Verification items for the finished model (mm, model axes). A direction names the side the tool comes from. Give positions to 0.01 mm unless a question says otherwise; leave off trailing zeros. Write each loop counter-clockwise with the first axis right and the second up, starting at its lowest first coordinate (ties: lowest second). Pieces come first, ordered by that corner, then holes. Notation, with made-up numbers: (15, 13.25) -> (40, 13.25) arc R18 ccw to (40, 41.25) -> close; hole circle Ø10 at (72, 69.5). An arc over 180 degrees is marked (long way). Answer as CSV lines item,"result". Start each with the question number.
1) Gauge pin test, flat ends, axial feed: pin 1 Ø4 at (x, z) = (69, 22) entering from +Y; pin 2 Ø15 at (y, z) = (-137, 0.5) entering from -X; pin 3 Ø3 at (x, z) = (-3.5, 20.5) entering from +Y. Record the tip position at first contact, or that the pin passes through.
2) Sectioned sample at B-B on x = 118. Record the cut outline in (y, z), and give its area (3 significant figures).
3) Sectioned sample at A-A on z = -4.5. Record the cut outline in (x, y), and give its area (3 significant figures).
4) Material ranges on L1, parallel to Z at x = 101.5, y = -80; L2, parallel to X at y = -132.5, z = 8.5; L3, parallel to Y at x = 132, z = -8, recorded low to high.
5) Mould release check, pull along Z, two halves, no side actions. Record for faces 4 (the flat face through (0, -125, 8)), 5 (the flat face through (73.95, -134.863, 25.056)), 6 (the flat face through (125, -5, 17)): released by +Z, released by -Z, zero draft, split by the parting line, or undercut.
6) Tool access check on faces 1 (the flat face through (84, -84, 0)), 2 (the flat face through (-2, -125, 19)), 3 (the flat face through (-2, -100, 21)). Record the directions out of +Z, -Z, +X, -X, +Y, -Y that give a thin tool (end or side, any length) a straight path to the whole face; none if there is none.
7) Sectioned sample at D-D on z = 7. Record the cut outline in (x, y), and give its area (3 significant figures).
8) Sectioned sample at C-C on y = -23.5. Record the cut outline in (x, z), and give its area (3 significant figures).
```python
from build123d import *

# Parameters (mm, degrees)
F1_DEPTH  = 29
F3_DEPTH  = 150
F5_DEPTH  = 150.001
F7_DEPTH  = 5
F9_DEPTH  = 5
F11_DEPTH = 150


with BuildPart() as f1:
    # F0 (on Top) → F1 (new body)
    with BuildSketch(Plane.XY):
        with BuildLine():
            Line((150, -150), (150, 0))
            Line((150, 0), (100, 0))
            ThreePointArc((100, 0), (70.7106781187, -70.7106781187), (0, -100))
            Line((0, -100), (0, -150))
            Line((0, -150), (150, -150))
        make_face()
    extrude(amount=F1_DEPTH)

    # F2 (on face) → F3 (cut, through all)
    with BuildSketch(Plane(origin=(0, 0, 0), x_dir=(0, -1, 0), z_dir=(-1, 0, 0))):
        Polygon((150, 29), (120.1435935394, 29), (150, 21), align=None)
    extrude(amount=-F3_DEPTH, mode=Mode.SUBTRACT)

    # F4 (on face) → F5 (cut, through all)
    with BuildSketch(Plane(origin=(0, 0, 0), x_dir=(-1, 0, 0), z_dir=(0, 1, 0))):
        Polygon((-120.1435935394, 29), (-150, 29), (-150, 21), align=None)
    extrude(amount=-F5_DEPTH, mode=Mode.SUBTRACT)

    # F6 (on face) → F7 (join)
    with BuildSketch(Plane(origin=(0, 0, 0), x_dir=(0, -1, 0), z_dir=(-1, 0, 0))):
        Polygon((150, 15), (100, 23), (100, 19), (150, 11), align=None)
    extrude(amount=F7_DEPTH)

    # F8 (on face) → F9 (cut)
    with BuildSketch(Plane(origin=(0, 0, 0), x_dir=(-1, 0, 0), z_dir=(0, 1, 0))):
        Polygon((-95.0627968404, 24.0399525055), (-100, 23.25), (-150, 15.25), (-150, 10.75), (-100, 18.75), (-95.0627968404, 19.5399525055), align=None)
    extrude(amount=-F9_DEPTH, mode=Mode.SUBTRACT)

    # F10 (on face) → F11 (join)
    with BuildSketch(Plane(origin=(0, 0, 0), x_dir=(0, -1, 0), z_dir=(-1, 0, 0))):
        Polygon((150, -11), (150, 0), (139, 0), align=None)
    extrude(amount=-F11_DEPTH)

    # F12 (on face) → F13 (join, up to the next surface of F1)
    with BuildSketch(Plane(origin=(0, 0, 0), x_dir=(-1, 0, 0), z_dir=(0, 1, 0))):
        Polygon((-139, 0), (-150, 0), (-150, -11), align=None)
    extrude(until=Until.NEXT, dir=(0, -1, 0))


solid = f1.part
```
Ans:
1,pin 1,"stops at y = -70.42"
1,pin 2,"stops at x = 0"
1,pin 3,"stops at y = -100"
2,outline,"(-150, -11) -> (-139, 0) -> (0, 0) -> (0, 15.87) -> (-5, 15.87) -> (-5, 20.37) -> (0, 20.37) -> (0, 29) -> (-120.14, 29) -> (-150, 21) -> close"
2,area,"4,270 mm²"
3,outline,"(0, -150) -> (150, -150) -> (150, 0) -> (143.5, 0) -> (143.5, -143.5) -> (0, -143.5) -> close"
3,area,"1,910 mm²"
4,L1,"z = 0 to 29"
4,L2,"x = 0 to 150"
4,L3,"y = -150 to -147"
5,face 4,"zero draft"
5,face 5,"released by +Z"
5,face 6,"undercut"
6,face 1,"-Z, -X, +Y"
6,face 2,"+Z, -X, -Y"
6,face 3,"+Z, -Z, -X, +Y"
7,outline,"(0, -150) -> (150, -150) -> (150, 0) -> (100, 0) arc R100 cw to (0, -100) -> close"
7,area,"14,600 mm²"
8,outline,"(97.2, 0) -> (139, 0) -> (150, -11) -> (150, 21) -> (120.14, 29) -> (97.2, 29) -> close"
8,area,"1,470 mm²"
